Source: CAD feature listing. Evaluate the final solid. Frame: model axes, mm. Face numbers are marked on the shaded views. A direction names the side the tool comes from. Give positions to 0.01 mm unless a question says otherwise; leave off trailing zeros. Write each loop counter-clockwise with the first axis right and the second up, starting at its lowest first coordinate (ties: lowest second). Pieces come first, ordered by that corner, then holes. Notation, with made-up numbers: (-24.5, -36) -> (29.5, -36) arc R20 ccw to (29.5, -17) -> close; hole circle Ø1 at (-7, 18.5). An arc over 180 degrees is marked (long way). Write item = value, one per line.
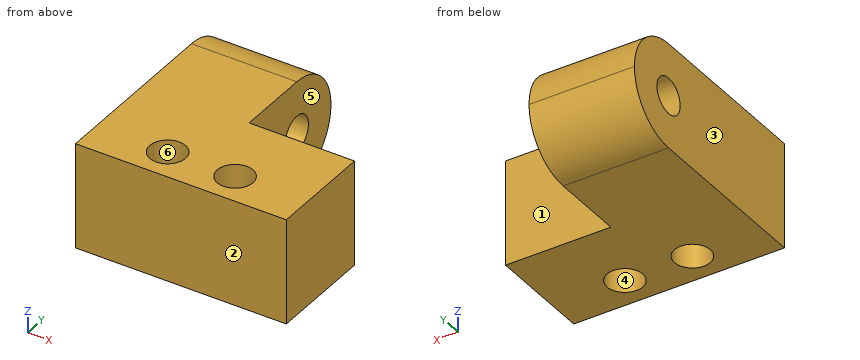
Autodesk Inventor part; units mm, degrees
ref_plane "YZ Plane" through (0, 0, 0) normal (1, 0, 0) x (0, 1, 0)
ref_plane "XZ Plane" through (0, 0, 0) normal (0, 1, 0) x (-1, 0, 0)
ref_plane "XY Plane" through (0, 0, 0) normal (0, 0, 1) x (1, 0, 0)
sketch "スケッチ4" plane through (0, 0, 0) normal (0, 0, 1) x (1, 0, 0)
  line L0 (0, 0) -> (20, 0)
  line L1 (20, 0) -> (20, 10)
  line L2 (0, 22) -> (0, 0)
  line L3 (0, 22) -> (10, 22)
  line L4 (10, 22) -> (10, 10)
  line L5 (10, 10) -> (20, 10)
  line L6 (10, 0) -> (10, 7.8024) construction
  circle A0 centre (6.8, 3) radius 1.7
  circle A1 centre (13.2, 3) radius 1.7
  dimension "d19" = 20
  dimension "d20" = 22
  dimension "d21" = 12
  dimension "d22" = 10
  dimension "d23" = 6.4
  dimension "d24" = 3.4
  dimension "d25" = 3
extrude "押し出し4" add sketch "スケッチ4" along normal blind 10
sketch "スケッチ5" plane through (0, 0, 0) normal (-1, 0, 0) x (0, 0, 1)
  line L0 (0, 22) -> (10, 22)
  line L1 (5, 22) -> (5, 17) construction
  circle A0 centre (5, 17) radius 1.7
  point P0 (0, 0)
  dimension "d28" = 3.4
  dimension "d29" = 5
extrude "押し出し5" cut sketch "スケッチ5" against normal blind 10
fillet "フィレット2" radius 5 2 edges at (5, 22, 0) (5, 22, 10)
properties part number "pixymount1"
(1) Access query for the marked faces 5 and 6. Directions: +Z, -Z, +X, -X, +Y, -Y. A direction counts if a zero-diameter tool reaches every point of the face in a straight line with its end or side. Return the directions, or none.
Values follow:
face_5 = +Z, -Z, +X, +Y
face_6 = +Z, -Z
(2) Pull-direction query (Y, two-part tool) for the marked faces 1, 2, 3 and 4; classes: pulls with the +Y half, pulls with the -Y half, needs draft (parallel to the pull), parting line crosses it, or undercut.
Values follow:
face_1 = pulls with the +Y half
face_2 = pulls with the -Y half
face_3 = needs draft
face_4 = undercut
(3) Section query B-B (x = 14). Return loops of the section in (y, z).
Values follow:
outline = (0, 0) -> (1.5, 0) -> (1.5, 10) -> (0, 10) -> close; (4.5, 0) -> (10, 0) -> (10, 10) -> (4.5, 10) -> close
(4) Material intervals for line 1 (Y direction, x = 13.2, z = 4.5); line 2 (X direction, y = 2.75, z = 8.5); line 3 (Y direction, x = 6.8, z = 5.75), sorted ascending.
Values follow:
line_1 = 0 to 1.3, 4.7 to 10
line_2 = 0 to 5.12, 8.48 to 11.52, 14.88 to 20
line_3 = 0 to 1.3, 4.7 to 15.47, 18.53 to 21.94
(5) Section query A-A (x = 6.8). Give the number of separate pieces and of enclosed holes in the cut face, plus the area to 3 significant figures.
Values follow:
separate_pieces = 2
enclosed_holes = 1
area = 166 mm2
(6) Section query C-C (z = 5.75). Return loops of the section in (x, y).
Values follow:
outline = (0, 0) -> (20, 0) -> (20, 10) -> (10, 10) -> (10, 15.47) -> (0, 15.47) -> close; (0, 18.53) -> (10, 18.53) -> (10, 21.94) -> (0, 21.94) -> close; hole circle Ø3.4 at (6.8, 3); hole circle Ø3.4 at (13.2, 3)
(7) First-contact query: pin 1 (4 mm diameter, centred on y = 14.5, z = 9, fed in from -X); pin 2 (5 mm diameter, centred on x = 17.5, z = 5.5, fed in from +Y); pin 3 (4 mm diameter, centred on y = 17, z = 5, fed in from +X). Flat tips, straight axial feed; report the tip coordinate or a pass-through.
Values follow:
pin_1 = 0
pin_2 = 10
pin_3 = 10
(8) Section query D-D (z = 3). Return loops of the section in (x, y), plus the area to 3 significant figures.
Values follow:
outline = (0, 0) -> (20, 0) -> (20, 10) -> (10, 10) -> (10, 21.58) -> (0, 21.58) -> close; hole circle Ø3.4 at (6.8, 3); hole circle Ø3.4 at (13.2, 3)
area = 298 mm2
